from build123d import *

# Parameters (mm, degrees)
F2_SIZE = 1
F3_R    = 1


with BuildPart() as f1:
    # F0 (on Front) → F1 (revolve)
    with BuildSketch(Plane.XZ):
        Polygon((-96.6734094576, 23.8900707406), (-96.6734094576, 4.8900707406), (-36.6734094576, 4.8900707406), (-36.6734094576, 13.3900707406), (-86.6734094576, 13.3900707406), (-86.6734094576, 23.8900707406), align=None)
    revolve(axis=Axis((-29.0751103312, 0, -26.1099292594), (1, 0, 0)))

    # F2
    f2_edges = [f1.edges().sort_by_distance(p)[0] for p in [
        (-36.673409, 0, -57.109929),
        (-36.673409, 0, -65.609929),
        (-96.673409, 0, -57.109929),
    ]]
    chamfer(f2_edges, length=F2_SIZE)

    # F3
    f3_edges = [f1.edges().sort_by_distance(p)[0] for p in [
        (-86.673409, 0, -65.609929),
    ]]
    fillet(f3_edges, radius=F3_R)


solid = f1.part
Read the model definition and answer for the solid it produces. Units are mm, in the model's axes. A direction names the side the tool comes from. Coordinates: 2 decimals unless noted, no trailing zeros. Order: outer loops, then holes, each group sorted by start corner. A loop starts at its lowest first (then second) coordinate and runs counter-clockwise, first axis right, second up. Notation, with made-up numbers: (39.25, -36.5) -> (86.25, -36.5) arc R8 ccw to (86.25, -24.5) -> close; hole circle Ø7 at (28.5, 41). An arc over 180 degrees is marked (long way). Answer as a JSON object with one key per item and string values.
1) Consider line 1 along Z through (x, y) = (-75, 0); line 2 along Y through (x, z) = (-91.5, 1); line 3 along X through (y, z) = (46.5, -36). Determine where each line is inside the solid, lowest interval first. Write a range as from..to.
Model answer:
{"line 1": "z = -65.61..-57.11, 4.89..13.39", "line 2": "y = -42.01..-15.04, 15.04..42.01", "line 3": "x = -96.67..-86.67"}
2) A cutting plane is placed at A-A, the plane y = 0. Determine the outline of the cut face in (x, z), plus the area to 3 significant figures.
Model answer:
{"outline": "(-96.67, -76.11) -> (-86.67, -76.11) -> (-86.67, -66.61) arc R1 cw to (-85.67, -65.61) -> (-37.67, -65.61) -> (-36.67, -64.61) -> (-36.67, -58.11) -> (-37.67, -57.11) -> (-95.67, -57.11) -> (-96.67, -58.11) -> close; (-96.67, 5.89) -> (-95.67, 4.89) -> (-37.67, 4.89) -> (-36.67, 5.89) -> (-36.67, 12.39) -> (-37.67, 13.39) -> (-85.67, 13.39) arc R1 cw to (-86.67, 14.39) -> (-86.67, 23.89) -> (-96.67, 23.89) -> close", "area": "1,230 mm²"}
3) A cutting plane is placed at B-B, the plane x = -91.5. Determine the outline of the cut face in (y, z).
Model answer:
{"outline": "circle Ø100 at (0, -26.11); hole circle Ø62 at (0, -26.11)"}
4) Each of these flat-tipped pins is pushed along its axis until it touches: pin 1 (4 mm diameter, centred on x = -73, z = -9, fed in from +Y); pin 2 (10 mm diameter, centred on x = -84, y = 33.5, fed in from -Z); pin 3 (1 mm diameter, centred on x = -86, y = -15, fed in from +Z). Where does it stop, or does it pass through?
Model answer:
{"pin 1": "stops at y = 36.5", "pin 2": "stops at z = -66.64", "pin 3": "stops at z = 10.93"}
5) A tool of negligible diameter and unlimited length cuts with its end or side. For faces 1 (the face through (-62.009, -11.865, 11.566)), 2 (the face through (-96.673, 33, -27)), from which of +Z, -Z, +X, -X, +Y, -Y can it reach the whole face along a straight path? Write none if from no direction.
Model answer:
{"face 1": "+X", "face 2": "+Z, -Z, -X, +Y, -Y"}
6) The mould has two halves that part along Y. Classify faces 3 (the face through (-36.673, -32, -32)), 4 (the face through (-66.27, -9.31, 3.46)), 5 (the face through (-91.74, -2.2, -76.06)): released by +Y, released by -Y, zero draft, split by the parting line, or undercut.
Model answer:
{"face 3": "zero draft", "face 4": "undercut", "face 5": "split by the parting line"}
7) A cutting plane is placed at C-C, the plane x = -55.5. Determine the outline of the cut face in (y, z).
Model answer:
{"outline": "circle Ø79 at (0, -26.11); hole circle Ø62 at (0, -26.11)"}
